```python
from build123d import *

# Parameters (mm, degrees)
F0_R     = 5
F1_DEPTH = 10
F2_DEPTH = 6


with BuildPart() as f1:
    # F0 (on Front) → F1 (new body, symmetric)
    with BuildSketch(Plane.XZ):
        with BuildLine():
            ThreePointArc((7, 192.858572), (9.219544, 196.127017), (10, 200))
            ThreePointArc((10, 200), (-3.872983, 209.219544), (-7, 192.858572))
            ThreePointArc((-7, 192.858572), (0, 190), (7, 192.858572))
        make_face()
        with Locations((0, 200)):
            Circle(F0_R, mode=Mode.SUBTRACT)
        with BuildLine():
            ThreePointArc((7, -192.858572), (0, -190), (-7, -192.858572))
            ThreePointArc((-7, -192.858572), (-3.872983, -209.219544), (10, -200))
            ThreePointArc((10, -200), (9.219544, -196.127017), (7, -192.858572))
        make_face()
        with Locations((0, -200)):
            Circle(F0_R, mode=Mode.SUBTRACT)
    extrude(amount=F1_DEPTH, both=True)

    # F0 (on Front) → F2 (join, symmetric)
    with BuildSketch(Plane.XZ):
        with BuildLine():
            ThreePointArc((7, 192.858572), (0, 190), (-7, 192.858572))
            Line((-7, 192.858572), (-7, -192.858572))
            ThreePointArc((-7, -192.858572), (0, -190), (7, -192.858572))
            Line((7, -192.858572), (7, 192.858572))
        make_face()
    extrude(amount=F2_DEPTH, both=True)


solid = f1.part
```
Can you work these out from the model? Positions are in its coordinate system, mm. A direction names the side the tool comes from. Give positions to 0.01 mm unless a question says otherwise; leave off trailing zeros. Loops run counter-clockwise (first coordinate to the right, second up) from the corner with the lowest first, then second, coordinate; pieces in that order, holes last. Notation, with made-up numbers: M 27,-5 L 64,-5 A28 cw 64,23 Z; hole C -29.75,42 d11. An arc over 180 degrees is marked long. One line per question, with ' | ' between items. Start each with the question number.
Q1. If we mould it in two halves opening along Z, with no side actions, what happens to faces 1 (the cylindrical face through (-0.651, 0.14, -195.043)), 2 (the flat face through (-5, 10, 198))? For each: +Z half, -Z half, draft (parallel to the pull), parting line (faces both ways), or undercut.
Q2. For pin 1 Ø8 at (y, z) = (7.5, 166.5) entering from -X; pin 2 Ø1 at (y, z) = (0, 132.5) entering from +X; pin 3 Ø4 at (x, z) = (5.5, 59) entering from -Y, each with a flat end and sliding along its axis, tell me the tip position at first contact or that it passes through.
Q3. If we section it at C-C (z = -5): Please give me the cut outline in (x, y), plus the area to 3 significant figures.
Q4. If we section it at A-A (x = 0): Please give me the cut outline in (y, z).
Q5. If we section it at B-B (y = 0.5): Please give me the cut outline in (x, z).
Q6. If I drill on line 1 (Z direction, x = 0, y = -4.75); line 2 (Z direction, x = -0.5, y = 9.25); line 3 (Z direction, x = -2, y = -3.25), over which ranges is the centre line in solid material (lowest first)? Write a range as from..to.
Q7. For faces 3 (the flat face through (-7, 0, 3)), 4 (the cylindrical face through (-0.651, 0.14, 204.957)), 5 (the flat face through (7, 0, -3)), 6 (the flat face through (0, 6, 3)), 7 (the flat face through (-5, -10, -202)), which set-ups out of +Z, -Z, +X, -X, +Y, -Y let a thin tool reach every point of the face, with its end or its side?
Computed:
1) face 1: undercut | face 2: draft
2) pin 1: stops at x = -7 | pin 2: stops at x = 7 | pin 3: stops at y = -6
3) outline: M -7,-6 L 7,-6 L 7,6 L -7,6 Z | area: 168 mm²
4) outline: M -10,-210 L 10,-210 L 10,-205 L -10,-205 Z; M -10,-195 L 10,-195 L 10,-190 L 6,-190 L 6,190 L 10,190 L 10,195 L -10,195 L -10,190 L -6,190 L -6,-190 L -10,-190 Z; M -10,205 L 10,205 L 10,210 L -10,210 Z
5) outline: M -7,-192.86 A10 ccw long 10,-200 A10 ccw 7,-192.86 L 7,192.86 A10 ccw 10,200 A10 ccw long -7,192.86 Z; hole C 0,-200 d10; hole C 0,200 d10
6) line 1: z = -210..-205, -195..195, 205..210 | line 2: z = -209.99..-204.97, -195.03..-190.01, 190.01..195.03, 204.97..209.99 | line 3: z = -209.8..-204.58, -195.42..195.42, 204.58..209.8
7) face 3: -X, +Y, -Y | face 4: +Y, -Y | face 5: +X, +Y, -Y | face 6: +X, -X, +Y | face 7: +Z, -Z, +X, -X, -Y
